Input: part model. Units: mm. Frame: model coordinates. A direction names the side the tool comes from. Give positions to 0.01 mm unless a question says otherwise; leave off trailing zeros. Loops run counter-clockwise (first coordinate to the right, second up) from the corner with the lowest first, then second, coordinate; pieces in that order, holes last. Notation, with made-up numbers: M -20,-25 L 4,-25 A19 cw 4,-10 Z; hole C -38,-1 d3. An arc over 180 degrees is marked long. Answer as a JSON object with one key per item and string values. Group by question number.
```python
from build123d import *

# Parameters (mm, degrees)
SKETCH1_W           = 254
SKETCH1_H           = 118.999
BOSS_EXTRUDE1_DEPTH = 38.1
SKETCH2_W           = 33.02
SKETCH2_H           = 104.775
CUT_EXTRUDE1_DEPTH  = 241.3
SKETCH5_W           = 238.017311759
SKETCH5_H           = 93.599
CUT_EXTRUDE2_DEPTH  = 38.354


with BuildPart() as part:
    # Sketch1 → Boss-Extrude1 (new body)
    with BuildSketch(Plane.XY):
        Rectangle(SKETCH1_W, SKETCH1_H)
    extrude(amount=-BOSS_EXTRUDE1_DEPTH)

    # Sketch2 → Cut-Extrude1 (cut)
    with BuildSketch(Plane.ZY.offset(127)):
        with Locations((-19.05, 0)):
            Rectangle(SKETCH2_W, SKETCH2_H)
    extrude(amount=-CUT_EXTRUDE1_DEPTH, mode=Mode.SUBTRACT)

    # Sketch5 → Cut-Extrude2 (cut)
    with BuildSketch(Plane.XY):
        with Locations((-7.991344121, 0)):
            Rectangle(SKETCH5_W, SKETCH5_H)
    extrude(amount=-CUT_EXTRUDE2_DEPTH, mode=Mode.SUBTRACT)


solid = part.part
```
1. Section C-C (z = -14.5). Output: boundary loops of the cut face in (x, y), then the cut area to 3 significant figures.
2. Section B-B (y = 17.5). Output: boundary loops of the cut face in (x, z), then the cut area to 3 significant figures.
3. Material intervals for L1, parallel to Y at x = -86, z = -11; L2, parallel to Z at x = 85, y = -47; L3, parallel to X at y = -1, z = -22, sorted ascending.
4. Mould query, pull axis Y, two halves, no side actions, for faces 1 (the flat face through (-2, 59.5, -19)), 2 (the flat face through (-7, -47, -2.54)), 3 (the flat face through (127, -1, -19)). Classes: pulls with the +Y half, pulls with the -Y half, needs draft (parallel to the pull), parting line crosses it, or undercut.
5. Section A-A (x = -31). Output: boundary loops of the cut face in (y, z), then the cut area to 3 significant figures.
6. Reachability of faces 4 (the flat face through (114.3, 1, -19)), 5 (the flat face through (-127, 54, -19)) from +Z, -Z, +X, -X, +Y, -Y: full face, straight path, thin tool, end or side. Return the list, or none.
7. First-contact query: P1, Ø1.3, axis at y = 3.5, z = -2, coming from the -X side; P2, Ø3, axis at y = 47, z = -4.5, coming from the -X side. Flat tips, straight axial feed; report the tip coordinate or a pass-through.
Geometry results:
{
 "1": {"outline": "M -127,-59.5 L 127,-59.5 L 127,59.5 L -127,59.5 L -127,52.39 L 114.3,52.39 L 114.3,-52.39 L -127,-52.39 Z", "area": "4,940 mm2"},
 "2": {"outline": "M 111.02,-38.1 L 127,-38.1 L 127,0 L 111.02,0 L 111.02,-2.54 L 114.3,-2.54 L 114.3,-35.56 L 111.02,-35.56 Z", "area": "501 mm2"},
 "3": {"L1": "-59.5 to -52.39, 52.39 to 59.5", "L2": "-38.1 to -35.56, -2.54 to 0", "L3": "114.3 to 127"},
 "4": {"face 1": "pulls with the +Y half", "face 2": "undercut", "face 3": "needs draft"},
 "5": {"outline": "M -59.5,-38.1 L -46.8,-38.1 L -46.8,-35.56 L -52.39,-35.56 L -52.39,-2.54 L -46.8,-2.54 L -46.8,0 L -59.5,0 Z; M 46.8,-38.1 L 59.5,-38.1 L 59.5,0 L 46.8,0 L 46.8,-2.54 L 52.39,-2.54 L 52.39,-35.56 L 46.8,-35.56 Z", "area": "599 mm2"},
 "6": {"face 4": "-X", "face 5": "+Z, -Z, -X, +Y, -Y"},
 "7": {"P1": "x = 111.02", "P2": "x = 114.3"}
}
